Can you work these out from the model? Positions are in its coordinate system, mm. Face numbers are marked on the shaded views. A direction names the side the tool comes from. Coordinates: 2 decimals unless noted, no trailing zeros. Loops run counter-clockwise (first coordinate to the right, second up) from the corner with the lowest first, then second, coordinate; pieces in that order, holes last. Notation, with made-up numbers: (12, -29) -> (22, -29) arc R17 ccw to (22, -19) -> close; hole circle Ø9 at (21.25, 61). An arc over 180 degrees is marked (long way). Put each result on its own line as item: value. Start each with the question number.
Item 1: Will these pins go through, and if not, where does the flat tip stop? P1, Ø1, axis at x = 20.5, y = 2, coming from the +Z side; P2, Ø3.5, axis at x = 29, z = 0.5, coming from the +Y side; P3, Ø4.5, axis at x = 27.5, z = 0.5, coming from the -Y side.
Item 2: For the marked faces 1, 2, 3 and 4, which set-ups out of +Z, -Z, +X, -X, +Y, -Y let a thin tool reach every point of the face, with its end or its side?
Item 3: If we section it at A-A on y = -1.75: Please give me the cut outline in (x, z), plus the area to 3 significant figures.
Item 4: Please list where these lines run through material, in increasing order: L1, parallel to Y at x = 30, z = 0; L2, parallel to Z at x = 32.5, y = 0; L3, parallel to X at y = -1.5, z = 2.75. Write a range as from..to.
Item 5: If we section it at B-B on x = 16.5: Please give me the cut outline in (y, z).
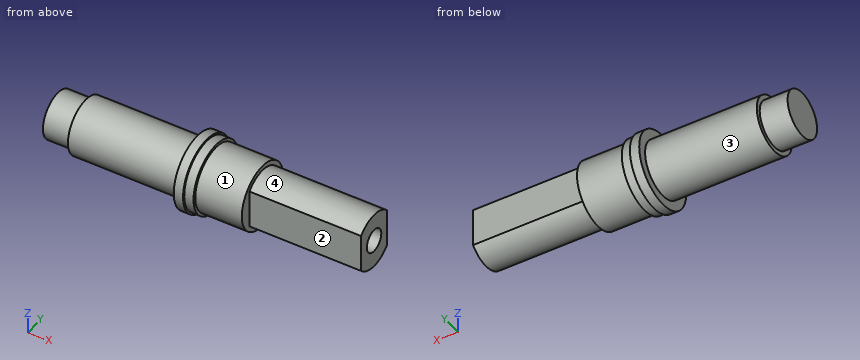
Autodesk Inventor part; units mm, degrees
ref_plane "YZ Plane" through (0, 0, 0) normal (1, 0, 0) x (0, 1, 0)
ref_plane "XZ Plane" through (0, 0, 0) normal (0, 1, 0) x (-1, 0, 0)
ref_plane "XY Plane" through (0, 0, 0) normal (0, 0, 1) x (1, 0, 0)
sketch "Sketch1" plane through (0, 0, 0) normal (0, 0, 1) x (1, 0, 0)
  line L0 (4, 3) -> (6, 3)
  line L1 (6, 3) -> (6, 3)
  line L2 (16.5, 3.5) -> (16.5, 3.5)
  line L3 (35, 3) -> (35, 0)
  line L4 (4, 3) -> (4, 2.5)
  line L5 (4, 2.5) -> (1, 2.5)
  line L6 (1, 2.5) -> (1, 0)
  line L7 (1, 0) -> (35, 0)
  line L8 (23, 3) -> (35, 3)
  line L9 (23, 3.5) -> (17, 3.5)
  line L10 (23, 3.5) -> (23, 3)
  line L11 (17, 3.5) -> (17, 4)
  line L12 (17, 4) -> (16, 4)
  line L13 (16, 4) -> (16, 3)
  line L14 (6, 3) -> (16, 3)
  point P0 (0, 0)
  dimension "d1" = 2
  dimension "d25" = 3
  dimension "d26" = 2.5
  dimension "d40" = 12
  dimension "d41" = 3
  dimension "d42" = 0.5
  dimension "d44" = 6
  dimension "d45" = 1
  dimension "d46" = 10
  dimension "d47" = 3
  dimension "d48" = 3
revolve "Revolution2" add sketch "Sketch1" angle 360 about axis through (1, 0, 0) along (1, 0, 0)
sketch "Sketch3" plane through (35, 0, 0) normal (1, 0, 0) x (0, 0, -1)
  circle A0 centre (0, 0) radius 3
  line L0 (-1.6583, 2.5) -> (1.6583, 2.5)
  line L1 (-1.6583, -2.5) -> (1.6583, -2.5)
  point P0 (0, 0)
  dimension "d21" = 0.5
  dimension "d31" = 0.5
extrude "Extrusion2" [suppressed]
sketch "Sketch4" plane through (4, 0, 0) normal (-1, 0, 0) x (0, 0, 1)
  line L0 (-1.6583, 2.5) -> (1.6583, 2.5)
  circle A0 centre (0, 0) radius 3
  line L1 (-1.6583, -2.5) -> (1.6583, -2.5)
  point P0 (0, 0)
  dimension "d27" = 0.5
  dimension "d30" = 0.5
extrude "Extrusion3" [suppressed]
sketch "Sketch5" plane through (35, 0, 0) normal (1, 0, 0) x (0, 0, -1)
  point P0 (0, 0)
  point P1 (0, 0)
hole "Hole1" at (35, 0, 0) direction (-1, 0, 0) diameter 2.459 depth 10 tip angle 118
sketch "Sketch6" plane through (35, 0, 0) normal (1, 0, 0) x (0, 0, -1)
  circle A0 centre (0, 0) radius 1.2295
  circle A1 centre (0, 0) radius 3
  circle A2 centre (0, 0) radius 3
  line L0 (-2.0396, 2.2) -> (2.0396, 2.2)
  line L1 (-2.0396, -2.2) -> (2.0396, -2.2)
  dimension "d56" = 2.2
  dimension "d57" = 2.2
extrude "Extrusion4" cut sketch "Sketch6" against normal up to surface (12 mm away) contours L0 A1 | A1 L1
sketch "Sketch7" plane through (17, 0, 0) normal (1, 0, 0) x (0, 0, -1)
  circle A0 centre (0, 0) radius 4
  circle A1 centre (0, 0) radius 3.5
  circle A2 centre (0, 0) radius 3.8
  point P0 (0, 0)
  dimension "d60" = 0.3
extrude "Extrusion5" add sketch "Sketch7" along normal blind 1 contours A2
properties part number "Wał koła" material "Aluminum 6061, Welded"
Solutions:
1. P1: z = 3.16
1. P2: y = 2.2
1. P3: y = -2.2
2. face 1: +X
2. face 2: +Z, -Z, +X, -Y
2. face 3: -X
2. face 4: +Z, +X
3. outline: (1, -1.79) -> (4, -1.79) -> (4, -2.44) -> (16, -2.44) -> (16, -3.6) -> (17, -3.6) -> (17, -3.37) -> (18, -3.37) -> (18, -3.03) -> (23, -3.03) -> (23, -2.44) -> (35, -2.44) -> (35, 2.44) -> (23, 2.44) -> (23, 3.03) -> (18, 3.03) -> (18, 3.37) -> (17, 3.37) -> (17, 3.6) -> (16, 3.6) -> (16, 2.44) -> (4, 2.44) -> (4, 1.79) -> (1, 1.79) -> close
3. area: 172 mm^2
4. L1: -2.2..-1.23, 1.23..2.2
4. L2: -3..-1.23, 1.23..3
4. L3: 16..23
5. outline: circle Ø8 at (0, 0)
